Build history of the part. All positions in model axes, mm. Face numbers are marked on the shaded views. Round coordinates to 2 decimals unless told otherwise and drop trailing zeros. Write each loop counter-clockwise with the first axis right and the second up, starting at its lowest first coordinate (ties: lowest second). Pieces come first, ordered by that corner, then holes. Notation, with made-up numbers: (19, 40) -> (47, 40) arc R36 cw to (47, 78) -> close; hole circle Ø1 at (44.25, 79). An arc over 180 degrees is marked (long way). One line per question, with ' | ' between items.
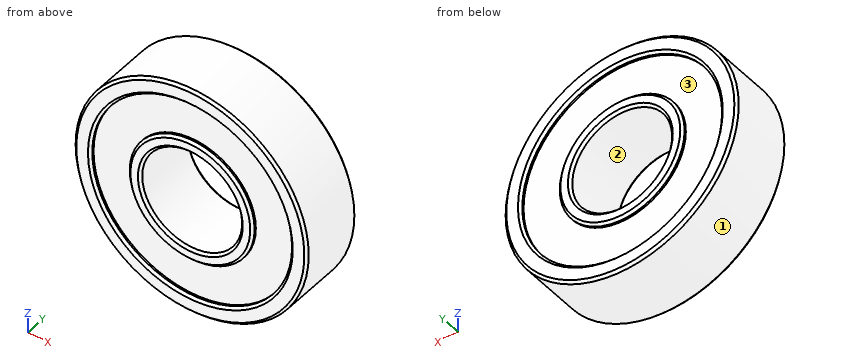
from build123d import *

# Parameters (mm, degrees)
CHAMFER1_SIZE = 0.3


with BuildPart() as part:
    # Sketch1 → Revolve1 (revolve)
    with BuildSketch(Plane.XY):
        Polygon((-6, 0), (-6, 8), (-7.5, 8), (-7.5, 7.5), (-12, 7.5), (-12, 8), (-14, 8), (-14, 0), (-12, 0), (-12, 0.5), (-7.5, 0.5), (-7.5, 0), align=None)
    revolve(axis=Axis((0, 0, 0), (0, 1, 0)))

    # Chamfer1
    chamfer1_edges = [part.edges().sort_by_distance(p)[0] for p in [
        (14, 0, 0),
        (14, 8, 0),
        (12, 8, 0),
        (7.5, 8, 0),
        (6, 8, 0),
        (6, 0, 0),
        (7.5, 0, 0),
        (12, 0, 0),
    ]]
    chamfer(chamfer1_edges, length=CHAMFER1_SIZE)


solid = part.part
(1) Wall check: line 1 (Z direction, x = 0, y = 7.6); line 2 (Z direction, x = 0, y = 2.75); line 3 (X direction, y = 1.5, z = 1). Give the ranges that are in metal, low to high. Write a range as from..to.
Calculated:
line 1: -14..-12, -7.5..-6, 6..7.5, 12..14 | line 2: -14..-6, 6..14 | line 3: -13.96..-5.92, 5.92..13.96
(2) Drop flat-ended pins along their axis: pin 1 (4 mm diameter, centred on y = 2, z = 1.5, fed in from -X); pin 2 (3 mm diameter, centred on y = 7, z = 10, fed in from -X); pin 3 (3 mm diameter, centred on x = -2.5, y = 7, fed in from +Z). Give the stop position or say it passes through.
Calculated:
pin 1: x = -14 | pin 2: x = -11.12 | pin 3: z = 13.96
(3) Slice it at A-A (y = 4.5). Write the cut outline in (x, z), then the cut area to 3 significant figures.
Calculated:
outline: circle Ø28 at (0, 0); hole circle Ø12 at (0, 0) | area: 503 mm2
(4) Mould opens along X. For the marked faces 1, 2 and 3 say: pulls with the +X half, pulls with the -X half, needs draft (parallel to the pull), parting line crosses it, or undercut.
Calculated:
face 1: parting line crosses it | face 2: undercut | face 3: undercut
